The model under review builds one solid part; all positions refer to its coordinate system, in mm. Face numbers are marked on the shaded views. A direction names the side the tool comes from. Coordinates: 2 decimals unless noted, no trailing zeros. Write each loop counter-clockwise with the first axis right and the second up, starting at its lowest first coordinate (ties: lowest second). Pieces come first, ordered by that corner, then holes. Notation, with made-up numbers: (79, -29.75) - (103, -29.75) arc R15 cw to (103, -12.75) - close; hole circle Ø6 at (61, 72). An arc over 180 degrees is marked (long way). Put each result on its own line as item: value.
Autodesk Inventor part; units mm, degrees
ref_plane "YZ Plane" through (0, 0, 0) normal (1, 0, 0) x (0, 1, 0)
ref_plane "XZ Plane" through (0, 0, 0) normal (0, 1, 0) x (-1, 0, 0)
ref_plane "XY Plane" through (0, 0, 0) normal (0, 0, 1) x (1, 0, 0)
sketch "Sketch1" plane through (0, 0, 0) normal (0, 0, 1) x (1, 0, 0)
  line L0 (-6.35, -25.4) -> (6.35, -25.4)
  line L1 (6.35, -25.4) -> (6.35, 25.4)
  line L2 (6.35, 25.4) -> (-6.35, 25.4)
  line L3 (-6.35, 25.4) -> (-6.35, -25.4)
  line L4 (-6.35, -25.4) -> (6.35, 25.4) construction
  line L5 (6.35, -25.4) -> (-6.35, 25.4) construction
  point P0 (0, 0)
  dimension "height" = 50.8
  dimension "width" = 12.7
extrude "Extrusion1" add sketch "Sketch1" against normal blind 12.7
sketch "Sketch3" plane through (0, 0, 0) normal (0, 0, 1) x (1, 0, 0)
  line L0 (-6.35, -9.525) -> (6.35, -9.525)
  line L1 (6.35, -9.525) -> (6.35, 9.525)
  line L2 (6.35, 9.525) -> (-6.35, 9.525)
  line L3 (-6.35, 9.525) -> (-6.35, -9.525)
  line L4 (-6.35, -9.525) -> (6.35, 9.525) construction
  line L5 (6.35, -9.525) -> (-6.35, 9.525) construction
  line L6 (6.35, 25.4) -> (-6.35, 25.4)
  point P0 (0, 0)
  dimension "Channel_Width" = 19.05
  dimension "d52" = 12.7
extrude "Extrusion3" add sketch "Sketch3" along normal blind 28.448
sketch "Sketch6" plane through (6.35, -25.4, -12.7) normal (1, 0, 0) x (0, 0, -1)
  line L0 (-12.7, 25.4) -> (-41.148, 25.4) construction
  line L1 (-41.148, 15.875) -> (-41.148, 34.925) construction
  line L2 (-12.7, 34.925) -> (-12.7, 50.8) construction
  point P0 (-26.924, 25.4)
  dimension "d53" = 14.224
hole "Hole5" at (6.35, 0, 14.224) direction (-1, 0, 0) diameter 3.9624 end through all
sketch "Sketch13" plane through (6.35, -25.4, -12.7) normal (1, 0, 0) x (0, 0, -1)
  line L0 (-12.7, 50.8) -> (0, 50.8)
  line L1 (0, 0) -> (-6.35, 0)
  line L2 (-6.35, 0) -> (-6.35, 50.8)
  line L3 (-6.35, 50.8) -> (0, 50.8)
  line L4 (0, 50.8) -> (0, 0)
  point P0 (-12.7, 25.4)
  dimension "d98" = 6.35
extrude "Extrusion5" cut sketch "Sketch13" against normal through all
sketch "Sketch14" plane through (-6.35, -25.4, 0) normal (-1, 0, 0) x (0, 0, 1)
  line L0 (0, 0) -> (-6.35, 0)
  line L1 (0, 0) -> (0, 15.875)
  line L2 (-6.35, 0) -> (0, 0)
  line L3 (0, 0) -> (0, 6.604)
  line L4 (0, 6.604) -> (-6.35, 6.604)
  line L5 (-6.35, 6.604) -> (-6.35, 0)
  point P0 (0, 25.4)
  dimension "d101" = 6.604
extrude "Extrusion6" cut sketch "Sketch14" against normal through all
sketch "Sketch16" plane through (6.35, 9.525, 0) normal (1, 0, 0) x (0, 0, -1)
  point P0 (0, -9.525)
sketch "Sketch17" plane through (0, 0, 0) normal (0, 0, 1) x (1, 0, 0)
  line L0 (-6.35, 25.4) -> (-6.35, 9.525)
  line L1 (-6.35, 9.525) -> (6.35, 9.525)
  line L2 (-6.35, 25.4) -> (6.35, 25.4)
  line L3 (6.35, 25.4) -> (6.35, 9.525)
  line L4 (6.35, 9.525) -> (-6.35, 9.525)
  line L5 (-6.35, 9.525) -> (-6.35, 25.4)
  point P0 (0, 0)
extrude "Extrusion7" cut sketch "Sketch17" against normal blind 0.381
sketch "Sketch18" plane through (0, 0, 0) normal (0, 0, 1) x (1, 0, 0)
  line L0 (-6.35, -18.796) -> (6.35, -18.796)
  line L1 (6.35, -9.525) -> (6.35, 9.525)
  line L2 (-6.35, -18.796) -> (6.35, -18.796)
  line L3 (6.35, -18.796) -> (6.35, -9.525)
  line L4 (6.35, -9.525) -> (-6.35, -9.525)
  line L5 (-6.35, -9.525) -> (-6.35, -18.796)
  point P0 (0, 0)
extrude "Extrusion8" cut sketch "Sketch18" against normal blind 0.381
sketch "Sketch10" plane through (0, 0, 28.448) normal (0, 0, 1) x (1, 0, 0)
  point P0 (0, 0)
sketch "Sketch12" plane through (-6.35, -9.525, 0) normal (0, -1, 0) x (1, 0, 0)
  point P0 (15.875, 15.875)
equation "\"width\" = partWidth"
equation "\"d52\" = width"
equation "\"Channel_Height\" = 2 * centerLineOfCylinder"
equation "\"partWidth\" = 12.7"
equation "\"centerLineOfCylinder\" = 14.224"
properties part number "vexTempConnectionToCylinder" material "Aluminum 6061"
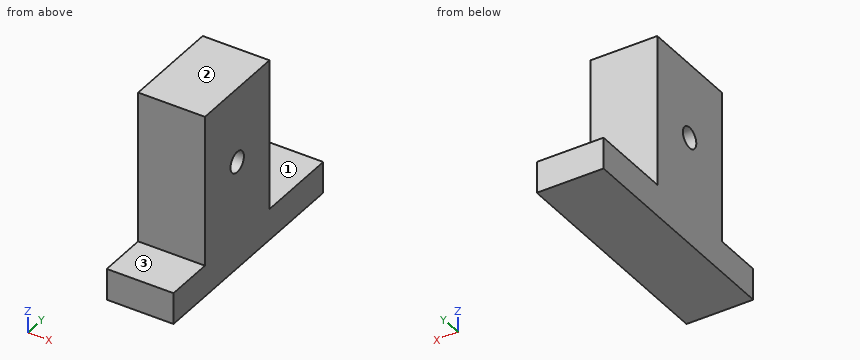
1. Machinability: for the marked faces 1, 2 and 3, which of the approach directions +Z, -Z, +X, -X, +Y, -Y give a long, thin tool a straight path to every point of the face, cutting with its end or side? Answer none if there is none.
Determined:
face 1: +Z, +X, -X, +Y
face 2: +Z, +X, -X, +Y, -Y
face 3: +Z, +X, -X, -Y
2. Consider section D-D on y = -11.5. State the section outline as (x, z) points, plus the area to 3 significant figures.
Determined:
outline: (-6.35, -6.35) - (6.35, -6.35) - (6.35, -0.38) - (-6.35, -0.38) - close
area: 75.8 mm^2
3. Consider section B-B on x = -0.25. State the section outline as (y, z) points (3 decimals), plus the area to 3 significant figures.
Determined:
outline: (-18.796, -6.35) - (25.4, -6.35) - (25.4, -0.381) - (9.525, -0.381) - (9.525, 28.448) - (-9.525, 28.448) - (-9.525, -0.381) - (-18.796, -0.381) - close; hole circle Ø3.962 at (0, 14.224)
area: 801 mm^2
4. Consider section C-C on z = 15.5. State the section outline as (x, y) points (3 decimals), plus the area to 3 significant figures.
Determined:
outline: (-6.35, -9.525) - (6.35, -9.525) - (6.35, -1.516) - (-6.35, -1.516) - close; (-6.35, 1.516) - (6.35, 1.516) - (6.35, 9.525) - (-6.35, 9.525) - close
area: 203 mm^2
5. Consider section A-A on y = 0. State the section outline as (x, z) points, plus the area to 3 significant figures.
Determined:
outline: (-6.35, -6.35) - (6.35, -6.35) - (6.35, 12.24) - (-6.35, 12.24) - close; (-6.35, 16.21) - (6.35, 16.21) - (6.35, 28.45) - (-6.35, 28.45) - close
area: 392 mm^2
6. For pin 1 Ø6 at (x, z) = (-4.5, 7) entering from +Y (3 decimals); pin 2 Ø4 at (x, y) = (-3, 15.5) entering from +Z; pin 3 Ø2.5 at (y, z) = (0, 14.224) entering from +X; pin 4 Ø5 at (x, z) = (-3.5, 11) entering from -Y (3 decimals), all flat-tipped, find the tip position at first contact; note any pin that passes through.
Determined:
pin 1: stops at y = 9.525
pin 2: stops at z = -0.38
pin 3: passes through
pin 4: stops at y = -9.525
7. To check wall thickness, follow probe 1 along Z at (x, y) = (0, 0); probe 2 along Z at (x, y) = (5.25, 23); probe 3 along Y at (x, z) = (3, 9.5) (3 decimals). State the ranges of each line that lie inside material, in increasing order.
Determined:
probe 1: z = -6.35 to 12.24, 16.21 to 28.45
probe 2: z = -6.35 to -0.38
probe 3: y = -9.525 to 9.525
